Autodesk Inventor part; units mm, degrees
ref_plane "YZ Plane" through (0, 0, 0) normal (1, 0, 0) x (0, 1, 0)
ref_plane "XZ Plane" through (0, 0, 0) normal (0, 1, 0) x (-1, 0, 0)
ref_plane "XY Plane" through (0, 0, 0) normal (0, 0, 1) x (1, 0, 0)
sketch "Schizzo3" plane through (0, 0, 0) normal (0, 1, 0) x (-1, 0, 0)
  line L0 (0, 0) -> (-2.5, 0)
  line L1 (-2.5, 0) -> (-2.5, -12)
  line L2 (-2.5, -12) -> (0, -12)
  line L3 (0, -12) -> (0, -9.2831)
  line L4 (0, -9.2831) -> (1.9415, -9.2831)
  line L5 (1.9415, -9.2831) -> (1.9415, -7.7495)
  line L6 (1.9415, -7.7495) -> (0, -7.7495)
  line L7 (0, -7.7495) -> (0, 0)
  line L8 (1.9415, -9.2831) -> (1.133, -9.9738)
  line L9 (1.133, -9.9738) -> (1.133, -9.2831)
  dimension "d5" = 2.5
  dimension "d6" = 12
revolve "Rivoluzione1" add sketch "Schizzo3" angle 360 about axis through (0, 0, 0) along (1, 0, 0)
fillet "Raccordo1" radius 2 1 edges at (2.5, 0, 12)
sketch "Schizzo6" plane through (0, 0, 0) normal (-1, 0, 0) x (0, 0, 1)
  point P0 (0, 0)
  point P1 (0, 0)
hole "Foro1" at (0, 0, 0) direction (1, 0, 0) diameter 4.5 depth 8 countersink diameter 7 countersink angle 90
Geometry check sheet. Reference: the model listing, model coordinates, mm. A direction names the side the tool comes from. Round coordinates to 2 decimals unless told otherwise and drop trailing zeros. Order: outer loops, then holes, each group sorted by start corner. A loop starts at its lowest first (then second) coordinate and runs counter-clockwise, first axis right, second up. Notation, with made-up numbers: M 18.25,-18.5 L 53.25,-18.5 A21 cw 53.25,-2.5 Z; hole C 67.25,54.25 d1. An arc over 180 degrees is marked long. Answer as CSV lines item,"result".
1) Gauge pin test, flat ends, axial feed: pin 1 Ø12.5 at (y, z) = (2, 3) entering from -X; pin 2 Ø5 at (y, z) = (0, 0) entering from -X. Record the tip position at first contact, or that the pin passes through.
Entries:
pin 1,"x = -1.94"
pin 2,"x = 1"
2) Sectioned sample at C-C on x = -0.35. Record the cut outline in (y, z).
Entries:
outline,"C 0,0 d18.57; hole C 0,0 d15.5"
3) Sectioned sample at D-D on x = 1.55. Record the cut outline in (y, z), and give its area (3 significant figures).
Entries:
outline,"C 0,0 d23.4; hole C 0,0 d4.5"
area,"414 mm2"
4) Mould release check, pull along X, two halves, no side actions. Record for faces 4 (the face through (-1.942, -8, 2)), 5 (the face through (0.25, -0.53, 11.99)), 6 (the face through (0, -9, -3)): +X half, -X half, draft (parallel to the pull), parting line (faces both ways), or undercut.
Entries:
face 4,"-X half"
face 5,"draft"
face 6,"undercut"
5) Tool access check on faces 1 (the face through (2.5, 2.4, 0.1)), 2 (the face through (0, -3.3, -1.6)), 3 (the face through (-0.574, 5.649, 7.367)). Record the directions out of +Z, -Z, +X, -X, +Y, -Y that give a thin tool (end or side, any length) a straight path to the whole face; none if there is none.
Entries:
face 1,"+Z, -Z, +X, +Y, -Y"
face 2,"-X"
face 3,"none"
6) Sectioned sample at A-A on z = 0. Record the cut outline in (x, y).
Entries:
outline,"M -1.94,-9.28 L -1.13,-9.97 L -1.13,-9.28 L 0,-9.28 L 0,-12 L 0.5,-12 A2 ccw 2.5,-10 L 2.5,-2.25 L 1.25,-2.25 L 0,-3.5 L 0,-7.75 L -1.94,-7.75 Z; M -1.94,7.75 L 0,7.75 L 0,3.5 L 1.25,2.25 L 2.5,2.25 L 2.5,10 A2 ccw 0.5,12 L 0,12 L 0,9.28 L -1.13,9.28 L -1.13,9.97 L -1.94,9.28 Z"
7) Thickness scan on probe 1 along Y at (x, z) = (-0.6, 0); probe 2 along X at (y, z) = (6.75, 1.5); probe 3 along Z at (x, y) = (1.4, -1). Record the ranges inside material, lowest first. Write a range as [from, to].
Entries:
probe 1,"[-9.28, -7.75], [7.75, 9.28]"
probe 2,"[0, 2.5]"
probe 3,"[-11.74, -2.02], [2.02, 11.74]"
